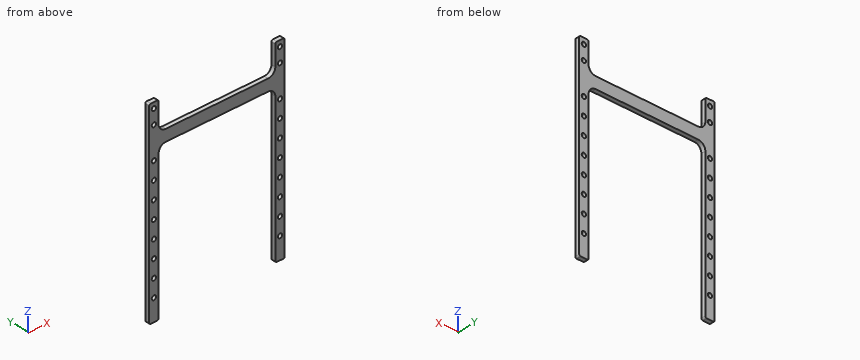
from build123d import *

# Parameters (mm, degrees)
BOSS_EXTRUDE1_DEPTH = 3
FILLET1_R           = 1
SKETCH2_R           = 1.5
CUT_EXTRUDE1_DEPTH  = 3


with BuildPart() as part:
    # Sketch1 → Boss-Extrude1 (new body)
    with BuildSketch(Plane(origin=(0, 0, 0), x_dir=(1, 0, 0), z_dir=(0, 1, 0))):
        with BuildLine():
            Line((-226.799741314, -52.674534602), (-233.299741314, -52.674534602))
            Line((-233.299741314, -52.674534602), (-233.299741314, 67.325465398))
            Line((-233.299741314, 67.325465398), (-233.299741314, 82.325465398))
            Line((-233.299741314, 82.325465398), (-226.799741314, 82.325465398))
            Line((-226.799741314, 82.325465398), (-226.799741314, 67.325465398))
            Line((-226.799741314, 67.325465398), (-226.799741314, -19.674534602))
            ThreePointArc((-226.799741314, -19.674534602), (-225.33527522, -23.210068508), (-221.799741314, -24.674534602))
            Line((-221.799741314, -24.674534602), (-150.799741314, -24.674534602))
            ThreePointArc((-150.799741314, -24.674534602), (-147.264207408, -23.210068508), (-145.799741314, -19.674534602))
            Line((-145.799741314, -19.674534602), (-145.799741314, 67.325465398))
            Line((-145.799741314, 67.325465398), (-145.799741314, 82.325465398))
            Line((-145.799741314, 82.325465398), (-139.299741314, 82.325465398))
            Line((-139.299741314, 82.325465398), (-139.299741314, 67.325465398))
            Line((-139.299741314, 67.325465398), (-139.299741314, -52.674534602))
            Line((-139.299741314, -52.674534602), (-145.799741314, -52.674534602))
            Line((-145.799741314, -52.674534602), (-145.799741314, -37.674534602))
            ThreePointArc((-145.799741314, -37.674534602), (-147.264207408, -34.139000697), (-150.799741314, -32.674534602))
            Line((-150.799741314, -32.674534602), (-221.799741314, -32.674534602))
            ThreePointArc((-221.799741314, -32.674534602), (-225.33527522, -34.139000697), (-226.799741314, -37.674534602))
            Line((-226.799741314, -37.674534602), (-226.799741314, -52.674534602))
        make_face()
    extrude(amount=BOSS_EXTRUDE1_DEPTH)

    # Fillet1
    fillet1_edges = [part.edges().sort_by_distance(p)[0] for p in [
        (-145.799741314, 1.5, -82.325465398),
        (-139.299741314, 1.5, -82.325465398),
        (-139.299741314, 1.5, 52.674534602),
        (-145.799741314, 1.5, 52.674534602),
        (-226.799741314, 1.5, 52.674534602),
        (-233.299741314, 1.5, 52.674534602),
        (-233.299741314, 1.5, -82.325465398),
        (-226.799741314, 1.5, -82.325465398),
    ]]
    fillet(fillet1_edges, radius=FILLET1_R)

    # Sketch2 → Cut-Extrude1 (cut)
    with BuildSketch(Plane(origin=(0, 3, 0), x_dir=(1, 0, 0), z_dir=(0, 1, 0))):
        with Locations((-230.049741314, 7.325465398)):
            Circle(SKETCH2_R)
        with Locations((-142.549741314, 7.325465398)):
            Circle(SKETCH2_R)
        with Locations((-230.049741314, 31.325465398)):
            Circle(SKETCH2_R)
        with Locations((-230.049741314, 55.325465398)):
            Circle(SKETCH2_R)
        with Locations((-230.049741314, 43.325465398)):
            Circle(SKETCH2_R)
        with Locations((-230.049741314, 19.325465398)):
            Circle(SKETCH2_R)
        with Locations((-230.049741314, -4.674534602)):
            Circle(SKETCH2_R)
        with Locations((-142.549741314, -4.674534602)):
            Circle(SKETCH2_R)
        with Locations((-230.049741314, -38.674534602)):
            Circle(SKETCH2_R)
        with Locations((-230.049741314, -48.674534602)):
            Circle(SKETCH2_R)
        with Locations((-142.549741314, -38.674534602)):
            Circle(SKETCH2_R)
        with Locations((-142.549741314, -48.674534602)):
            Circle(SKETCH2_R)
        with Locations((-142.549741314, 19.325465398)):
            Circle(SKETCH2_R)
        with Locations((-142.549741314, 31.325465398)):
            Circle(SKETCH2_R)
        with Locations((-142.549741314, 43.325465398)):
            Circle(SKETCH2_R)
        with Locations((-142.549741314, 55.325465398)):
            Circle(SKETCH2_R)
        with Locations((-230.049741314, -16.674534602)):
            Circle(SKETCH2_R)
        with Locations((-142.549741314, -16.674534602)):
            Circle(SKETCH2_R)
        with Locations((-230.049741314, 67.325465398)):
            Circle(SKETCH2_R)
        with Locations((-142.549741314, 67.325465398)):
            Circle(SKETCH2_R)
    extrude(amount=-CUT_EXTRUDE1_DEPTH, mode=Mode.SUBTRACT)


solid = part.part
Model file for the job. Use its own axes, mm. Round coordinates to 2 decimals unless told otherwise and drop trailing zeros. Loops run counter-clockwise (first coordinate to the right, second up) from the corner with the lowest first, then second, coordinate; pieces in that order, holes last. Notation, with made-up numbers: (-13, 63) - (22, 63) arc R17 cw to (22, 69) - close; hole circle Ø5 at (44, 29.5). An arc over 180 degrees is marked (long way). Write each question's results on one line, items separated by ' | '.
(1) Saw through at A-A, the plane z = 42.5. List the corners of the cut face in (x, y).
Answer below:
outline: (-233.3, 0) - (-226.8, 0) - (-226.8, 3) - (-233.3, 3) - close; (-145.8, 0) - (-139.3, 0) - (-139.3, 3) - (-145.8, 3) - close
(2) Pin check, flat tips, straight feed: pin 1 (1.5 mm diameter, centred on x = -189, y = 1.5, fed in from +Z); pin 2 (1 mm diameter, centred on x = -184.5, y = 2, fed in from -Z). Stop position of each tip, or through.
Answer below:
pin 1: stops at z = 32.67 | pin 2: stops at z = 24.67
(3) Wall check: L1, parallel to X at y = 0.1, z = -7.5; L2, parallel to X at y = 2.3, z = -75.5; L3, parallel to Z at x = -181, y = 1.7. Give the ranges that are in metal, low to high.
Answer below:
L1: x = -233.3 to -231.54, -228.56 to -226.8, -145.8 to -144.04, -141.06 to -139.3 | L2: x = -233.3 to -226.8, -145.8 to -139.3 | L3: z = 24.67 to 32.67
(4) Saw through at C-C, the plane y = 1.6. Count the separate pieces of the cut face and the enclosed holes in it, then the cut area to 3 significant figures.
Answer below:
separate pieces: 1 | enclosed holes: 20 | area: 2,280 mm^2
(5) Saw through at B-B, the plane x = -183.5. List the corners of the cut face in (y, z), then the cut area to 3 significant figures.
Answer below:
outline: (0, 24.67) - (3, 24.67) - (3, 32.67) - (0, 32.67) - close | area: 24.0 mm^2
